Build history of the part. All positions in model axes, mm. Give positions to 0.01 mm unless a question says otherwise; leave off trailing zeros. Loops run counter-clockwise (first coordinate to the right, second up) from the corner with the lowest first, then second, coordinate; pieces in that order, holes last. Notation, with made-up numbers: (21, 69.5) -> (29, 69.5) arc R10 cw to (29, 78.5) -> close; hole circle Ø5 at (71.25, -12.5). An arc over 180 degrees is marked (long way). Answer in a Markdown table with one row per item. Add a question column.
from build123d import *


with BuildPart() as part:
    # Sketch2 → Revolve-Thin1 (revolve)
    with BuildSketch(Plane.XY):
        with BuildLine():
            ThreePointArc((10, 0), (0, 10), (-10, 0))
            Line((-10, 0), (-20, 0))
            ThreePointArc((-20, 0), (0, 20), (20, 0))
            Line((20, 0), (10, 0))
        make_face()
    revolve(axis=Axis((-10, 0, 0), (1, 0, 0)))

    # Sketch3 → Revolve-Thin2 (revolve)
    with BuildSketch(Plane.XY):
        Polygon((15, 0), (15, 11.417573163), (75, 11.417573163), (75, 0), (65, 0), (65, 1.417573163), (25, 1.417573163), (25, 0), align=None)
    revolve(axis=Axis((15, 0, 0), (1, 0, 0)))


solid = part.part
(1) Saw through at D-D, the plane y = -7.5. List the corners of the cut face in (x, z).
(2) Saw through at C-C, the plane x = 68. List the corners of the cut face in (y, z).
(3) Saw through at A-A, the plane y = 0. List the corners of the cut face in (x, z), then the cut area to 3 significant figures.
(4) Flat gauge pins, fed straight in: pin 1 Ø1.5 at (x, z) = (46, -0.5) entering from -Y; pin 2 Ø6 at (y, z) = (-14.5, 11) entering from -X; pin 3 Ø4 at (x, y) = (65.5, 2.5) entering from +Z. Where does each tip first touch, or does it go through?
(5) Wall check: line 1 along Z through (x, y) = (55.5, 0); line 2 along Y through (x, z) = (33.5, 5.5); line 3 along Z through (x, y) = (-4.5, 2). Give the ranges that are in metal, low to high. Write a range as from..to.
(6) Two-plate mould, pull along X, no slides. Class faces 1 (the flat face through (75, 0, 0)), 2 (the cylindrical face through (46.12, -2.475, -11.146)), 3 (the cylindrical face through (44.72, 0.65, -1.26)): released by +X, released by -X, zero draft, split by the parting line, or undercut.
Worked answers:
| question | item | result |
|---|---|---|
| 1 | outline | (16.42, -8.61) -> (75, -8.61) -> (75, 8.61) -> (16.42, 8.61) arc R18.54 ccw (long way) to start; hole circle Ø13.23 at (0, 0) |
| 2 | outline | circle Ø22.84 at (0, 0) |
| 3 | outline | (16.42, -11.42) -> (75, -11.42) -> (75, 11.42) -> (16.42, 11.42) arc R20 ccw (long way) to start; hole circle Ø20 at (0, 0); hole (25, -1.42) -> (65, -1.42) -> (65, 1.42) -> (25, 1.42) -> close |
| 3 | area | 2,110 mm^2 |
| 4 | pin 1 | y = -11.42 |
| 4 | pin 2 | x = -13 |
| 4 | pin 3 | z = 11.41 |
| 5 | line 1 | -11.42..-1.42, 1.42..11.42 |
| 5 | line 2 | -10.01..10.01 |
| 5 | line 3 | -19.38..-8.7, 8.7..19.38 |
| 6 | face 1 | released by +X |
| 6 | face 2 | zero draft |
| 6 | face 3 | undercut |
